Could you check a few things on this model? Use its own coordinates, in mm. Face numbers are marked on the shaded views. A direction names the side the tool comes from. Round coordinates to 2 decimals unless told otherwise and drop trailing zeros. Loops run counter-clockwise (first coordinate to the right, second up) from the corner with the lowest first, then second, coordinate; pieces in that order, holes last. Notation, with made-up numbers: (85, 35.5) -> (138, 35.5) arc R26 ccw to (138, 59.5) -> close; hole circle Ø1 at (-18.75, -35.5). An arc over 180 degrees is marked (long way). One line per item, written item: value.
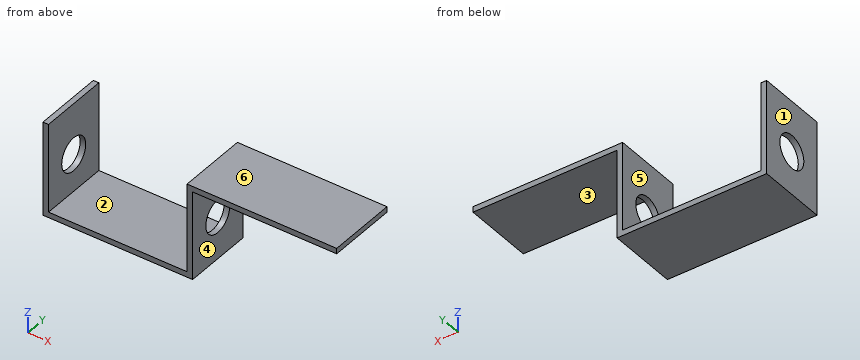
```python
from build123d import *

# Parameters (mm, degrees)
BOSS_EXTRUDE1_DEPTH = 80.01
SKETCH2_R           = 19.05
CUT_EXTRUDE1_DEPTH  = 175.768


with BuildPart() as part:
    # Sketch1 → Boss-Extrude1 (new body)
    with BuildSketch(Plane(origin=(0, 0, 0), x_dir=(1, 0, 0), z_dir=(0, 1, 0))):
        Polygon((85.725, 0), (85.725, 101.6), (-85.725, 101.6), (-85.725, -6.35), (-79.375, -6.35), (-79.375, 95.25), (79.375, 95.25), (79.375, -6.35), (110.08813222, -6.35), (250.825, -6.35), (250.825, 0), align=None)
    extrude(amount=BOSS_EXTRUDE1_DEPTH)

    # Sketch2 → Cut-Extrude1 (cut)
    with BuildSketch(Plane(origin=(85.725, 0, 0), x_dir=(0, 0, -1), z_dir=(1, 0, 0))):
        with Locations((52.214904531, 40.005)):
            Circle(SKETCH2_R)
    extrude(amount=-CUT_EXTRUDE1_DEPTH, mode=Mode.SUBTRACT)


solid = part.part
```
(1) Imagine slicing it at B-B on y = 51. Write out the boundary of the cut face in (x, z) (3 decimals).
Results below:
outline: (-85.725, -101.6) -> (85.725, -101.6) -> (85.725, -67.772) -> (79.375, -67.772) -> (79.375, -95.25) -> (-79.375, -95.25) -> (-79.375, -67.772) -> (-85.725, -67.772) -> close; (-85.725, -36.658) -> (-79.375, -36.658) -> (-79.375, 6.35) -> (-85.725, 6.35) -> close; (79.375, -36.658) -> (85.725, -36.658) -> (85.725, 0) -> (250.825, 0) -> (250.825, 6.35) -> (79.375, 6.35) -> close
(2) Imagine slicing it at A-A on z = -7.5. Write out the boundary of the cut face in (x, y) (3 decimals).
Results below:
outline: (-85.725, 0) -> (-79.375, 0) -> (-79.375, 80.01) -> (-85.725, 80.01) -> close; (79.375, 0) -> (85.725, 0) -> (85.725, 80.01) -> (79.375, 80.01) -> close
(3) On a 3-axis mill with a long thin cutter (end or side, diameter ignored), from which of +Z, -Z, +X, -X, +Y, -Y can I reach the whole of each face in a straight line? I mean the marked faces 1, 2 and 3. Say none if no direction works.
Results below:
face 1: +Z, -Z, -X, +Y, -Y
face 2: +Z, +Y, -Y
face 3: -Z, +X, +Y, -Y
(4) Please list where these lines run through material, in increasing order: L1, parallel to X at y = 50.5, z = -85 (3 decimals); L2, parallel to Z at x = -44, y = 35; L3, parallel to Z at x = 123.5, y = 9.
Results below:
L1: x = -85.725 to -79.375, 79.375 to 85.725
L2: z = -101.6 to -95.25
L3: z = 0 to 6.35
(5) Imagine slicing it at C-C on y = 9.5. Write out the boundary of the cut face in (x, z) (3 decimals), then the cut area to 3 significant figures.
Results below:
outline: (-85.725, -101.6) -> (85.725, -101.6) -> (85.725, 0) -> (250.825, 0) -> (250.825, 6.35) -> (79.375, 6.35) -> (79.375, -95.25) -> (-79.375, -95.25) -> (-79.375, 6.35) -> (-85.725, 6.35) -> close
area: 3,430 mm²
(6) We'd pull the mould along X, two halves only. Please class the marked faces 4, 5 and 6: +X half, -X half, draft (parallel to the pull), parting line (faces both ways), or undercut.
Results below:
face 4: +X half
face 5: undercut
face 6: draft
(7) For pin 1 Ø24 at (x, y) = (-31.5, 25.5) entering from +Z; pin 2 Ø1 at (y, z) = (39, -69) entering from +X; pin 3 Ø24 at (y, z) = (20, -69.5) entering from +X (3 decimals), each with a flat end and sliding along its axis, tell me the tip position at first contact or that it passes through.
Results below:
pin 1: stops at z = -95.25
pin 2: passes through
pin 3: stops at x = 85.725
(8) Imagine slicing it at D-D on z = -52. Write out the boundary of the cut face in (x, y) (3 decimals).
Results below:
outline: (-85.725, 0) -> (-79.375, 0) -> (-79.375, 20.956) -> (-85.725, 20.956) -> close; (-85.725, 59.054) -> (-79.375, 59.054) -> (-79.375, 80.01) -> (-85.725, 80.01) -> close; (79.375, 0) -> (85.725, 0) -> (85.725, 20.956) -> (79.375, 20.956) -> close; (79.375, 59.054) -> (85.725, 59.054) -> (85.725, 80.01) -> (79.375, 80.01) -> close
